Design review of the part built by this model. Coordinates are the model's own, in mm. A direction names the side the tool comes from. Round coordinates to 2 decimals unless told otherwise and drop trailing zeros. Loops run counter-clockwise (first coordinate to the right, second up) from the corner with the lowest first, then second, coordinate; pieces in that order, holes last. Notation, with made-up numbers: (-17.75, 59) -> (31.25, 59) arc R26 ccw to (31.25, 91) -> close; hole circle Ø6 at (79.5, -31). An arc over 180 degrees is marked (long way). Answer as CSV lines item,"result". Start each with the question number.
(1) To check wall thickness, follow line 1 (Z direction, x = 9.25, y = 7); line 2 (Y direction, x = 0, z = 9.5); line 3 (Y direction, x = 2.5, z = 4). State the ranges of each line that lie inside material, in increasing order. Write a range as from..to.
(2) Take a section at B-B, the plane x = 10.25. Write out the cut boundary in (y, z), and give its area (3 significant figures).
(3) Machinability: for faces 1 (the face through (0, -17.5, -3)), 2 (the face through (0, -14.5, -8)), 3 (the face through (0, -9, -5)), 4 (the face through (-1.46, -6.59, 5.93)), which of the approach directions +Z, -Z, +X, -X, +Y, -Y give a long, thin tool a straight path to every point of the face, cutting with its end or side? Answer none if there is none.
(4) Draft analysis for pull direction Z (two halves, no side actions). For faces 5 (the face through (-6.3, -2.9, 11)), 6 (the face through (0, -15, 0.5)), 7 (the face through (4.125, -13, -5)), 8 (the face through (-6.3, -2.9, 1)), state which applies: +Z half, -Z half, draft (parallel to the pull), parting line (faces both ways), or undercut.
(5) Take a section at D-D, the plane x = 0. Write out the cut boundary in (y, z).
(6) For P1, Ø1, axis at x = -11, y = -7.5, coming from the -Z side; P2, Ø1.7, axis at x = -1.5, y = -15, coming from the -Z side; P3, Ø7.5, axis at x = 0, y = 0, coming from the -Z side; P4, Ø2, axis at y = -12, z = -2, coming from the -X side (3 decimals), all flat-tipped, find the tip position at first contact; note any pin that passes through.
(7) Take a section at C-C, the plane z = 6.25. Write out the cut boundary in (x, y).
(8) Take a section at A-A, the plane y = 0. Write out the cut boundary in (x, z).
from build123d import *

# Parameters (mm, degrees)
SKETCH_1_R           = 13.8
SKETCH_1_R_2         = 6.25
EXTRUDE_1_DEPTH      = 1
SKETCH_2_R           = 6.75
SKETCH_2_R_2         = 6.25
EXTRUDE_2_DEPTH      = 10
SKETCH_3_R           = 13.8
SKETCH_3_R_2         = 6.25
EXTRUDE_3_DEPTH      = 1
EXTRUDE_4_DEPTH      = 7
EXTRUDE_4_DEPTH_BACK = 0.5
SKETCH_4_W           = 8.25
SKETCH_4_H           = 8.5
SKETCH_5_W           = 8.25
SKETCH_5_H           = 5.5
EXTRUDE_5_DEPTH      = 3.2
FILLET_1_R           = 0.3


with BuildPart() as part:
    # Эскиз1 → Бобышка-Вытянуть1 (new body)
    with BuildSketch(Plane.XY):
        Circle(SKETCH_1_R)
        Circle(SKETCH_1_R_2, mode=Mode.SUBTRACT)
    extrude(amount=EXTRUDE_1_DEPTH)

    # Эскиз2 → Бобышка-Вытянуть2 (add)
    with BuildSketch(Plane.XY.offset(1)):
        Circle(SKETCH_2_R)
        Circle(SKETCH_2_R_2, mode=Mode.SUBTRACT)
    extrude(amount=EXTRUDE_2_DEPTH)

    # Эскиз3 → Бобышка-Вытянуть3 (add)
    with BuildSketch(Plane.XY.offset(11)):
        Circle(SKETCH_3_R)
        Circle(SKETCH_3_R_2, mode=Mode.SUBTRACT)
    extrude(amount=EXTRUDE_3_DEPTH)

    # Эскиз4 → Бобышка-Вытянуть4 (add, two sides: drawn at the far end of the back side and taken through both)
    with BuildSketch(Plane(origin=(0, 0, 0), x_dir=(-1, 0, 0), z_dir=(0, 0, -1)).offset(-EXTRUDE_4_DEPTH_BACK)):
        with Locations((0, -13.25)):
            Rectangle(SKETCH_4_W, SKETCH_4_H)
    extrude(amount=EXTRUDE_4_DEPTH + EXTRUDE_4_DEPTH_BACK)

    # Эскиз5 → Бобышка-Вытянуть5 (add)
    with BuildSketch(Plane(origin=(0, 0, -7), x_dir=(-1, 0, 0), z_dir=(0, 0, -1))):
        with Locations((0, -11.75)):
            Rectangle(SKETCH_5_W, SKETCH_5_H)
    extrude(amount=EXTRUDE_5_DEPTH)

    # Скругление1
    fillet_1_edges = [part.edges().sort_by_distance(p)[0] for p in [
        (4.125, -9, -5.1),
        (-4.125, -9, -5.1),
        (4.125, -14.5, -8.6),
        (-4.125, -14.5, -8.6),
        (4.125, -11.75, -10.2),
        (0, -14.5, -10.2),
        (-4.125, -11.75, -10.2),
        (0, -9, -10.2),
    ]]
    fillet(fillet_1_edges, radius=FILLET_1_R)


solid = part.part
The answers:
1,line 1,"0..1, 11..12"
1,line 2,"-6.75..-6.25, 6.25..6.75"
1,line 3,"-6.27..-5.73, 5.73..6.27"
2,outline,"(-9.24, 0) -> (9.24, 0) -> (9.24, 1) -> (-9.24, 1) -> close; (-9.24, 11) -> (9.24, 11) -> (9.24, 12) -> (-9.24, 12) -> close"
2,area,"37.0 mm²"
3,face 1,"+Z, -Z, +X, -X, -Y"
3,face 2,"-Z, +X, -X, -Y"
3,face 3,"-Z, +X, -X, +Y"
3,face 4,"none"
4,face 5,"undercut"
4,face 6,"+Z half"
4,face 7,"draft"
4,face 8,"undercut"
5,outline,"(-17.5, -7) -> (-14.5, -7) -> (-14.5, -9.9) arc R0.3 ccw to (-14.2, -10.2) -> (-9.3, -10.2) arc R0.3 ccw to (-9, -9.9) -> (-9, 0) -> (-6.25, 0) -> (-6.25, 12) -> (-13.8, 12) -> (-13.8, 11) -> (-6.75, 11) -> (-6.75, 1) -> (-13.8, 1) -> (-13.8, 0.5) -> (-17.5, 0.5) -> close; (6.25, 0) -> (13.8, 0) -> (13.8, 1) -> (6.75, 1) -> (6.75, 11) -> (13.8, 11) -> (13.8, 12) -> (6.25, 12) -> close"
6,P1,"z = 0"
6,P2,"z = -10.2"
6,P3,"through"
6,P4,"x = -4.125"
7,outline,"circle Ø13.5 at (0, 0); hole circle Ø12.5 at (0, 0)"
8,outline,"(-13.8, 0) -> (-6.25, 0) -> (-6.25, 12) -> (-13.8, 12) -> (-13.8, 11) -> (-6.75, 11) -> (-6.75, 1) -> (-13.8, 1) -> close; (6.25, 0) -> (13.8, 0) -> (13.8, 1) -> (6.75, 1) -> (6.75, 11) -> (13.8, 11) -> (13.8, 12) -> (6.25, 12) -> close"
